Verification items for the finished model (mm, model axes). Give positions to 0.01 mm unless a question says otherwise; leave off trailing zeros. Order: outer loops, then holes, each group sorted by start corner. A loop starts at its lowest first (then second) coordinate and runs counter-clockwise, first axis right, second up.
(1) Sectioned sample at A-A on x = -56. Record the cut outline in (y, z).
(2) Gauge pin test, flat end, axial feed: pin 1 (3.5 mm diameter, centred on x = -25, y = 25, fed in from +Z). Record the tip position at first contact, or that the pin passes through.
(3) Scan lines: L1, parallel to X at y = -25.5, z = 0.75; L2, parallel to Y at x = 25, z = 2; L3, parallel to Y at x = 68.5, z = 4. Record each from-to range of solid material in increasing order.
```python
from build123d import *

# Parameters (mm, degrees)
SKETCH1_W           = 336
SKETCH1_H           = 78
SKETCH1_R           = 2.1
BOSS_EXTRUDE1_DEPTH = 8
CUT_EXTRUDE1_REACH  = 338
SKETCH2_R           = 1.8


with BuildPart() as part:
    # Sketch1 → Boss-Extrude1 (new body)
    with BuildSketch(Plane.XY):
        Rectangle(SKETCH1_W, SKETCH1_H)
        with Locations((-25, 25)):
            Circle(SKETCH1_R, mode=Mode.SUBTRACT)
        with Locations((25, 25)):
            Circle(SKETCH1_R, mode=Mode.SUBTRACT)
        with Locations((25, -25)):
            Circle(SKETCH1_R, mode=Mode.SUBTRACT)
        with Locations((-25, -25)):
            Circle(SKETCH1_R, mode=Mode.SUBTRACT)
    extrude(amount=BOSS_EXTRUDE1_DEPTH)

    # Sketch2 → Cut-Extrude1 (cut, up to next)
    with BuildSketch(Plane(origin=(168, 0, 0), x_dir=(0, 0, -1), z_dir=(1, 0, 0)), mode=Mode.PRIVATE) as cut_extrude1_sk1:
        with Locations((-4, 33)):
            Circle(SKETCH2_R)
    cut_extrude1_tool1 = extrude(cut_extrude1_sk1.sketch, amount=-CUT_EXTRUDE1_REACH, mode=Mode.PRIVATE) & part.part
    add(cut_extrude1_tool1.solids().sort_by_distance((168, 33, 4))[0], mode=Mode.SUBTRACT)
    # Sketch2 → Cut-Extrude1 (cut, up to next)
    with BuildSketch(Plane(origin=(168, 0, 0), x_dir=(0, 0, -1), z_dir=(1, 0, 0)), mode=Mode.PRIVATE) as cut_extrude1_sk2:
        with Locations((-4, 7)):
            Circle(SKETCH2_R)
    cut_extrude1_tool2 = extrude(cut_extrude1_sk2.sketch, amount=-CUT_EXTRUDE1_REACH, mode=Mode.PRIVATE) & part.part
    add(cut_extrude1_tool2.solids().sort_by_distance((168, 7, 4))[0], mode=Mode.SUBTRACT)
    # Sketch2 → Cut-Extrude1 (cut, up to next)
    with BuildSketch(Plane(origin=(168, 0, 0), x_dir=(0, 0, -1), z_dir=(1, 0, 0)), mode=Mode.PRIVATE) as cut_extrude1_sk3:
        with Locations((-4, -7)):
            Circle(SKETCH2_R)
    cut_extrude1_tool3 = extrude(cut_extrude1_sk3.sketch, amount=-CUT_EXTRUDE1_REACH, mode=Mode.PRIVATE) & part.part
    add(cut_extrude1_tool3.solids().sort_by_distance((168, -7, 4))[0], mode=Mode.SUBTRACT)
    # Sketch2 → Cut-Extrude1 (cut, up to next)
    with BuildSketch(Plane(origin=(168, 0, 0), x_dir=(0, 0, -1), z_dir=(1, 0, 0)), mode=Mode.PRIVATE) as cut_extrude1_sk4:
        with Locations((-4, -33)):
            Circle(SKETCH2_R)
    cut_extrude1_tool4 = extrude(cut_extrude1_sk4.sketch, amount=-CUT_EXTRUDE1_REACH, mode=Mode.PRIVATE) & part.part
    add(cut_extrude1_tool4.solids().sort_by_distance((168, -33, 4))[0], mode=Mode.SUBTRACT)


solid = part.part
```
Ans:
1. outline: (-39, 0) - (39, 0) - (39, 8) - (-39, 8) - close; hole circle Ø3.6 at (-33, 4); hole circle Ø3.6 at (-7, 4); hole circle Ø3.6 at (7, 4); hole circle Ø3.6 at (33, 4)
2. pin 1: passes through
3. L1: x = -168 to -27.04, -22.96 to 22.96, 27.04 to 168
3. L2: y = -39 to -27.1, -22.9 to 22.9, 27.1 to 39
3. L3: y = -39 to -34.8, -31.2 to -8.8, -5.2 to 5.2, 8.8 to 31.2, 34.8 to 39
